Geometry: final body of the model. Coordinates: model frame, mm. Face numbers are marked on the shaded views. A direction names the side the tool comes from. Coordinates: 2 decimals unless noted, no trailing zeros. Order: outer loops, then holes, each group sorted by start corner. A loop starts at its lowest first (then second) coordinate and runs counter-clockwise, first axis right, second up. Notation, with made-up numbers: M -13,87 L 17,87 A24 ccw 17,115 Z; hole C 67,35 d2. An arc over 180 degrees is marked long. Use CSV: the item, a comma, the result in double quotes. Start each with the question number.
Q1. Access query for the marked faces 5, 6, 7, 8 and 9. Directions: +Z, -Z, +X, -X, +Y, -Y. A direction counts if a zero-diameter tool reaches every point of the face in a straight line with its end or side. Return the directions, or none.
Q2. Section query C-C, the plane y = 16.25. State how many separate pieces and enclosed holes the cut face has, and give its area (3 significant figures).
Q3. Mould query, pull axis Y, two halves, no side actions, for the marked faces 1, 2, 3 and 4. Classes: +Y half, -Y half, draft (parallel to the pull), parting line (faces both ways), or undercut.
Q4. First-contact query: P1, Ø3, axis at x = -11, y = 3, coming from the -Z side; P2, Ø1.4, axis at x = -22, y = 22, coming from the -Z side; P3, Ø4, axis at y = -0.5, z = 0.5, coming from the -X side. Flat tips, straight axial feed; report the tip coordinate or a pass-through.
Q5. Ray query, probe 1 along Y at (x, z) = (20, 25.5); probe 2 along X at (y, z) = (-6, 26); probe 3 along Y at (x, z) = (0, 25.65). Return the intervals inside material, ascending.
Q6. Section query B-B, the plane y = 0. Output: boundary loops of the cut face in (x, z).
Q7. Section query D-D, the plane x = 5. Output: boundary loops of the cut face in (y, z), and give its area (3 significant figures).
Q8. Section query A-A, the plane z = 11. Output: boundary loops of the cut face in (x, y), and give its area (3 significant figures).
from build123d import *
from build123d.topology import SkipClean

# Parameters (mm, degrees)
SKETCH1_R               = 35.25
SKETCH1_R_2             = 31.25
BOSS_EXTRUDE1_DEPTH     = 7.5
CUT_EXTRUDE1_DEPTH      = 51.412052
BOSS_EXTRUDE2_DEPTH     = 15
BOSS_EXTRUDE3_DEPTH     = 5
CUT_EXTRUDE2_START      = -10
SKETCH8_R               = 2.25
CUT_EXTRUDE2_DEPTH      = 97.386619
CUT_EXTRUDE3_START      = -10
CUT_EXTRUDE3_DEPTH      = 12.5
MIRROR3_START           = -10
MIRROR3_COPY_1_SKETCH_R = 2.25
MIRROR3_COPY_1_DEPTH    = 97.386619
MIRROR3_COPY_2_DEPTH    = 12.5
CUT_EXTRUDE4_DEPTH      = 62.638425
CUT_EXTRUDE4_DEPTH_BACK = 62.638425
FILLET1_R               = 5
SKETCH11_R              = 2.25
EXAMPLE_MOUNT_DEPTH     = 62.638425
FILLET2_R               = 1


with BuildPart() as part:
    # Sketch1 → Boss-Extrude1 (new, symmetric)
    with BuildSketch(Plane.XY):
        Circle(SKETCH1_R)
        Circle(SKETCH1_R_2, mode=Mode.SUBTRACT)
    extrude(amount=BOSS_EXTRUDE1_DEPTH, both=True)

    # Sketch2 → Cut-Extrude1 (cut, symmetric)
    with BuildSketch(Plane.XY):
        with BuildLine():
            Line((20.218569, 28.87511), (17.924264, 25.598501))
            ThreePointArc((17.924264, 25.598501), (0, 31.25), (-17.924264, 25.598501))
            Line((-17.924264, 25.598501), (-20.218569, 28.87511))
            ThreePointArc((-20.218569, 28.87511), (0, 35.25), (20.218569, 28.87511))
        make_face()
    cut_extrude1 = extrude(amount=CUT_EXTRUDE1_DEPTH, both=True, mode=Mode.SUBTRACT)

    # Mirror1: Cut-Extrude1 across plane
    add(cut_extrude1.mirror(Plane.ZX), mode=Mode.SUBTRACT)

    # Sketch3 → Boss-Extrude2 (add)
    with SkipClean():  # the faces are left unmerged after this step: merging them gives an invalid solid
        with BuildSketch(Plane.XY.offset(7.5)):
            with BuildLine():
                Line((-17.924264, 25.598501), (-22.512875, 32.151718))
                ThreePointArc((-22.512875, 32.151718), (-39.25, 0), (-22.512875, -32.151718))
                Line((-22.512875, -32.151718), (-17.924264, -25.598501))
                ThreePointArc((-17.924264, -25.598501), (-31.25, 0), (-17.924264, 25.598501))
            make_face()
            with BuildLine():
                Line((17.924264, -25.598501), (22.512875, -32.151718))
                ThreePointArc((22.512875, -32.151718), (39.25, 0), (22.512875, 32.151718))
                Line((22.512875, 32.151718), (17.924264, 25.598501))
                ThreePointArc((17.924264, 25.598501), (31.25, 0), (17.924264, -25.598501))
            make_face()
        extrude(amount=BOSS_EXTRUDE2_DEPTH)

    # Sketch4 → Boss-Extrude3 (add)
    with SkipClean():  # the faces are left unmerged after this step: merging them gives an invalid solid
        with BuildSketch(Plane.XY.offset(22.5)):
            with BuildLine():
                Line((22.512875, 32.151718), (-22.512875, 32.151718))
                ThreePointArc((-22.512875, 32.151718), (-39.25, 0), (-22.512875, -32.151718))
                Line((-22.512875, -32.151718), (22.512875, -32.151718))
                ThreePointArc((22.512875, -32.151718), (39.25, 0), (22.512875, 32.151718))
            make_face()
        extrude(amount=BOSS_EXTRUDE3_DEPTH)

    # Sketch8 → Cut-Extrude2 (cut)
    with SkipClean():  # the faces are left unmerged after this step: merging them gives an invalid solid
        with BuildSketch(Plane(origin=(22.097087, 22.097087, 0), x_dir=(0.7071067811865486, -0.7071067811865465, 0), z_dir=(0.7071067811865465, 0.7071067811865486, 0)).offset(CUT_EXTRUDE2_START)):
            with Locations(Location((0, 0, 0), (0, 0, 180))):
                Circle(SKETCH8_R)
        cut_extrude2 = extrude(amount=CUT_EXTRUDE2_DEPTH, mode=Mode.SUBTRACT)

    # Sketch9 → Cut-Extrude3 (cut)
    with SkipClean():  # the faces are left unmerged after this step: merging them gives an invalid solid
        with BuildSketch(Plane(origin=(22.097087, 22.097087, 0), x_dir=(0.7071067811865486, -0.7071067811865465, 0), z_dir=(0.7071067811865465, 0.7071067811865486, 0)).offset(CUT_EXTRUDE3_START)):
            Polygon((2.020726, -3.5), (4.041452, 0), (2.020726, 3.5), (-2.020726, 3.5), (-4.041452, 0), (-2.020726, -3.5), align=None)
        cut_extrude3 = extrude(amount=CUT_EXTRUDE3_DEPTH, mode=Mode.SUBTRACT)

    # Mirror2: Cut-Extrude2, Cut-Extrude3 across plane
    with SkipClean():  # the faces are left unmerged after this step: merging them gives an invalid solid
        add(cut_extrude2.mirror(Plane.ZX), mode=Mode.SUBTRACT)
        add(cut_extrude3.mirror(Plane.ZX), mode=Mode.SUBTRACT)

    # Mirror3: Cut-Extrude2, Cut-Extrude3 across plane
    with SkipClean():  # the faces are left unmerged after this step: merging them gives an invalid solid
        add(cut_extrude2.mirror(Plane(origin=(0, 0, 0), x_dir=(0, 0, 1), z_dir=(1, 0, 0))), mode=Mode.SUBTRACT)
        add(cut_extrude3.mirror(Plane(origin=(0, 0, 0), x_dir=(0, 0, 1), z_dir=(1, 0, 0))), mode=Mode.SUBTRACT)

    # Mirror3 copy 1 sketch → Mirror3 copy 1 (cut)
    with SkipClean():  # the faces are left unmerged after this step: merging them gives an invalid solid
        with BuildSketch(Plane(origin=(-22.097087, -22.097087, 0), x_dir=(-0.7071067811865486, 0.7071067811865465, 0), z_dir=(-0.7071067811865465, -0.7071067811865486, 0)).offset(MIRROR3_START)):
            with Locations(Location((0, 0, 0), (0, 0, 180))):
                Circle(MIRROR3_COPY_1_SKETCH_R)
        extrude(amount=MIRROR3_COPY_1_DEPTH, mode=Mode.SUBTRACT)

    # Mirror3 copy 2 sketch → Mirror3 copy 2 (cut)
    with SkipClean():  # the faces are left unmerged after this step: merging them gives an invalid solid
        with BuildSketch(Plane(origin=(-22.097087, -22.097087, 0), x_dir=(-0.7071067811865486, 0.7071067811865465, 0), z_dir=(-0.7071067811865465, -0.7071067811865486, 0)).offset(MIRROR3_START)):
            Polygon((2.020726, -3.5), (4.041452, 0), (2.020726, 3.5), (-2.020726, 3.5), (-4.041452, 0), (-2.020726, -3.5), align=None)
        extrude(amount=MIRROR3_COPY_2_DEPTH, mode=Mode.SUBTRACT)

    # Sketch10 → Cut-Extrude4 (cut, two sides: drawn at the far end of the back side and taken through both)
    with SkipClean():  # the faces are left unmerged after this step: merging them gives an invalid solid
        with BuildSketch(Plane.XY.offset(27.5).offset(-CUT_EXTRUDE4_DEPTH_BACK)):
            with BuildLine():
                Line((-22.512875, -32.151718), (-7.169705, -10.239401))
                ThreePointArc((-7.169705, -10.239401), (0, 12.5), (7.169705, -10.239401))
                Line((7.169705, -10.239401), (22.512875, -32.151718))
                Line((22.512875, -32.151718), (-22.512875, -32.151718))
            make_face()
        extrude(amount=CUT_EXTRUDE4_DEPTH + CUT_EXTRUDE4_DEPTH_BACK, mode=Mode.SUBTRACT)

    # Fillet1
    fillet1_edges = [part.edges().sort_by_distance(p)[0] for p in [
        (-7.169705, -10.239401, 25),
        (7.169705, -10.239401, 25),
    ]]
    fillet(fillet1_edges, radius=FILLET1_R)

    # Sketch11 → example_mount (cut, through all)
    with SkipClean():  # the faces are left unmerged after this step: merging them gives an invalid solid
        with BuildSketch(Plane.XY.offset(27.5)):
            with Locations((-20, -6.25)):
                Circle(SKETCH11_R)
            with Locations((-20, 16.25)):
                Circle(SKETCH11_R)
            with Locations((20, 16.25)):
                Circle(SKETCH11_R)
            with Locations((20, -6.25)):
                Circle(SKETCH11_R)
        extrude(amount=-EXAMPLE_MOUNT_DEPTH, mode=Mode.SUBTRACT)

    # Fillet2
    fillet2_edges = [part.edges().sort_by_distance(p)[0] for p in [
        (-31.25, 0, -7.5),
        (31.25, 0, -7.5),
    ]]
    fillet(fillet2_edges, radius=FILLET2_R)


solid = part.part
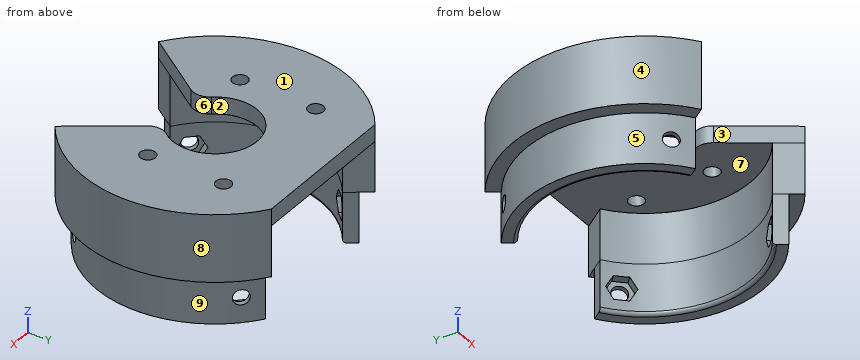
Responses:
1,face 5,"-Z, -X"
1,face 6,"+Z, -Z"
1,face 7,"-Z"
1,face 8,"+Z, -Z, +X"
1,face 9,"-Z, +X"
2,separate pieces,"3"
2,enclosed holes,"0"
2,area,"720 mm²"
3,face 1,"draft"
3,face 2,"undercut"
3,face 3,"-Y half"
3,face 4,"parting line"
4,P1,"stops at z = 22.5"
4,P2,"stops at z = -7.4"
4,P3,"stops at x = -35.25"
5,probe 1,"y = -28.56 to -8.5, -4 to 14, 18.5 to 32.15"
5,probe 2,"x = -38.79 to -22.24, -17.76 to -10.97, 10.97 to 17.76, 22.24 to 38.79"
5,probe 3,"y = 12.5 to 32.15"
6,outline,"M -39.25,7.5 L -35.25,7.5 L -35.25,-7.5 L -32.25,-7.5 A1 ccw -31.25,-6.5 L -31.25,22.5 L -12.5,22.5 L -12.5,27.5 L -39.25,27.5 Z; M 12.5,22.5 L 31.25,22.5 L 31.25,-6.5 A1 ccw 32.25,-7.5 L 35.25,-7.5 L 35.25,7.5 L 39.25,7.5 L 39.25,27.5 L 12.5,27.5 Z"
7,outline,"M 11.46,22.5 L 32.15,22.5 L 32.15,27.5 L 11.46,27.5 Z"
7,area,"103 mm²"
8,outline,"M -22.51,-32.15 L -17.92,-25.6 A31.25 cw -17.92,25.6 L -22.51,32.15 A39.25 ccw Z; M 17.92,-25.6 L 22.51,-32.15 A39.25 ccw 22.51,32.15 L 17.92,25.6 A31.25 cw Z"
8,area,"1,080 mm²"
